from build123d import *

# Parameters (mm, degrees)
SKETCH1_R           = 260
SKETCH1_R_2         = 250
EXTRUDE_THIN1_DEPTH = 2000
BOSS_EXTRUDE1_START = 1990
SKETCH1_2_R         = 250
BOSS_EXTRUDE1_DEPTH = 10
SKETCH1_3_R         = 250
BOSS_EXTRUDE2_DEPTH = 10


with BuildPart() as part:
    # Sketch1 → Extrude-Thin1 (new body)
    with BuildSketch(Plane(origin=(0, 0, 0), x_dir=(0, 0, -1), z_dir=(1, 0, 0))):
        Circle(SKETCH1_R)
        Circle(SKETCH1_R_2, mode=Mode.SUBTRACT)
    extrude(amount=EXTRUDE_THIN1_DEPTH)

    # Sketch1<2> → Boss-Extrude1 (add)
    with BuildSketch(Plane(origin=(0, 0, 0), x_dir=(0, 0, -1), z_dir=(1, 0, 0)).offset(BOSS_EXTRUDE1_START)):
        Circle(SKETCH1_2_R)
    extrude(amount=BOSS_EXTRUDE1_DEPTH)

    # Sketch1<3> → Boss-Extrude2 (add)
    with BuildSketch(Plane(origin=(0, 0, 0), x_dir=(0, 0, -1), z_dir=(1, 0, 0))):
        Circle(SKETCH1_3_R)
    extrude(amount=BOSS_EXTRUDE2_DEPTH)


solid = part.part
Read the model definition and answer for the solid it produces. Units are mm, in the model's axes. A direction names the side the tool comes from. Round coordinates to 2 decimals unless told otherwise and drop trailing zeros. Write each loop counter-clockwise with the first axis right and the second up, starting at its lowest first coordinate (ties: lowest second). Pieces come first, ordered by that corner, then holes. Notation, with made-up numbers: (10, 18) - (30, 18) arc R35 cw to (30, 54) - close; hole circle Ø5 at (28, 81.5). An arc over 180 degrees is marked (long way). Use a Markdown table: item, result.
(1) Each of these flat-tipped pins is pushed along its axis until it touches: pin 1 Ø4 at (x, y) = (1278.5, -152) entering from +Z; pin 2 Ø2 at (x, z) = (1624.5, -157.5) entering from -Y; pin 3 Ø10 at (x, z) = (895.5, -201) entering from +Y. Where does it stop, or does it pass through?
Reported:
| item | result |
|---|---|
| pin 1 | z = 212.37 |
| pin 2 | y = -207.62 |
| pin 3 | y = 170.83 |
(2) Straight lines are drawn through the part: line 1 along Y through (x, z) = (812, 0); line 2 along X through (y, z) = (193, -29.5); line 3 along Z through (x, y) = (1105, -12). For each, find the intervals that lie inside material, in ascending order. Write a range as [from, to].
Reported:
| item | result |
|---|---|
| line 1 | [-260, -250], [250, 260] |
| line 2 | [0, 10], [1990, 2000] |
| line 3 | [-259.72, -249.71], [249.71, 259.72] |
(3) The mould has two halves that part along Y. Classify faces 3 (the cylindrical face through (986, 78.097, -247.994)), 4 (the flat face through (10, 4, 3)), 5 (the flat face through (0, 4, 4)): released by +Y, released by -Y, zero draft, split by the parting line, or undercut.
Reported:
| item | result |
|---|---|
| face 3 | split by the parting line |
| face 4 | undercut |
| face 5 | zero draft |
(4) The part is cut by section C-C (x = 1661.5). Write down the section's boundary in (y, z), then the cut area to 3 significant figures.
Reported:
| item | result |
|---|---|
| outline | circle Ø520 at (0, 0); hole circle Ø500 at (0, 0) |
| area | 16,000 mm2 |
(5) The part is cut by section A-A (y = 0). Write down the section's boundary in (x, z).
Reported:
| item | result |
|---|---|
| outline | (0, -260) - (2000, -260) - (2000, 260) - (0, 260) - close; hole (10, -250) - (1990, -250) - (1990, 250) - (10, 250) - close |
(6) Which of the six approach directions +Z, -Z, +X, -X, +Y, -Y give full straight-line access (tool end or side, diameter ignored) to faces 1 (the flat face through (2000, 4, 4)), 2 (the cylindrical face through (986.14, 10.99, 249.76))?
Reported:
| item | result |
|---|---|
| face 1 | +Z, -Z, +X, +Y, -Y |
| face 2 | none |
